Autodesk Inventor part; units mm, degrees
ref_plane "YZ Plane" through (0, 0, 0) normal (1, 0, 0) x (0, 1, 0)
ref_plane "XZ Plane" through (0, 0, 0) normal (0, 1, 0) x (-1, 0, 0)
ref_plane "XY Plane" through (0, 0, 0) normal (0, 0, 1) x (1, 0, 0)
sketch "Sketch9" plane through (0, 0, 0) normal (0, 1, 0) x (-1, 0, 0)
  line L0 (25, 25) -> (-25, 25)
  line L1 (-25, 25) -> (-25, -25)
  line L2 (-25, -25) -> (25, -25)
  line L3 (25, -25) -> (25, 25)
  line L4 (25, 25) -> (-25, -25) construction
  line L5 (-25, 25) -> (25, -25) construction
  line L6 (-23, 23) -> (23, 23)
  line L7 (23, 23) -> (23, -23)
  line L8 (23, -23) -> (-23, -23)
  line L9 (-23, -23) -> (-23, 23)
  point P0 (0, 0)
  dimension "d172" = 50
  dimension "d173" = 50
  dimension "d174" = 2
extrude "Extrusion3" add sketch "Sketch9" against normal blind 930
sketch "Sketch10" plane through (0, 0, 0) normal (1, 0, 0) x (0, 1, 0)
  line L0 (0, 25) -> (0, -25) construction
  line L1 (0, 25) -> (-930, 25) construction
  line L2 (-930, -25) -> (-930, 25) construction
  line L3 (0, -25) -> (-930, -25) construction
  line L4 (-925, 8.5) -> (-908, 8.5)
  line L5 (-908, 8.5) -> (-908, -8.5)
  line L6 (-908, -8.5) -> (-925, -8.5)
  line L7 (-925, -8.5) -> (-925, 8.5)
  line L8 (-925, 8.5) -> (-908, -8.5) construction
  line L9 (-908, 8.5) -> (-925, -8.5) construction
  circle A0 centre (-916.5, 0) radius 8.5
  line L10 (0, 25) -> (0, -25)
  point P0 (0, 0)
  point P1 (0, 0)
  point P2 (-930, 0)
  dimension "d177" = 17
  dimension "d178" = 17
  dimension "d191" = 5
extrude "Extrusion4" cut sketch "Sketch10" along normal through all contours A0
pattern_linear "Rectangular Pattern4" count 8 spacing 125 along (0, 1, 0) of "Extrusion4"
properties part number "TKS 3535 FDS WAY tube5" material "Stainless Steel"
Source: CAD feature listing. Evaluate the final solid. Frame: model axes, mm. A direction names the side the tool comes from. Give positions to 0.01 mm unless a question says otherwise; leave off trailing zeros. Loops run counter-clockwise (first coordinate to the right, second up) from the corner with the lowest first, then second, coordinate; pieces in that order, holes last. Notation, with made-up numbers: (68.5, 85.5) -> (122.5, 85.5) arc R8 cw to (122.5, 97.5) -> close; hole circle Ø5 at (14, 37.25). An arc over 180 degrees is marked (long way). Use a Markdown table: item, result. Add a question column.
1) Pull-direction query (Z, two-part tool) for faces 4 (the face through (2, 0, -24)), 5 (the face through (0, -458, 23)), 6 (the face through (0, -458, -25)); classes: +Z half, -Z half, draft (parallel to the pull), parting line (faces both ways), or undercut.
2) Reachability of faces 1 (the face through (24, -550, 0)), 2 (the face through (2, -930, -24)), 3 (the face through (0, -458, -23)) from +Z, -Z, +X, -X, +Y, -Y: full face, straight path, thin tool, end or side. Return the list, or none.
3) Line query: line 1 along Z through (x, y) = (-11, -457); line 2 along Z through (x, y) = (24.25, -416.5). Output: solid intervals per line, ascending. Write a range as [from, to].
4) Section query B-B, the plane y = -273.5. Return the cut outline in (x, z).
5) Section query C-C, the plane y = -666.5. Return the cut outline in (x, z), then the cut area to 3 significant figures.
6) Section query D-D, the plane z = 0. Count the separate pieces of the cut face and the enclosed holes in it, then the cut area to 3 significant figures.
7) Section query A-A, the plane x = -1. Return the cut outline in (y, z), then the cut area to 3 significant figures.
Numbers:
| question | item | result |
|---|---|---|
| 1 | face 4 | draft |
| 1 | face 5 | undercut |
| 1 | face 6 | -Z half |
| 2 | face 1 | +X |
| 2 | face 2 | +Z, -Z, +X, -X, -Y |
| 2 | face 3 | +Y, -Y |
| 3 | line 1 | z = [-25, -23], [23, 25] |
| 3 | line 2 | z = [-25, -8.5], [8.5, 25] |
| 4 | outline | (-25, -25) -> (25, -25) -> (25, 25) -> (-25, 25) -> close; hole (-23, -23) -> (23, -23) -> (23, 23) -> (-23, 23) -> close |
| 5 | outline | (-25, -25) -> (25, -25) -> (25, -8.5) -> (23, -8.5) -> (23, -23) -> (-23, -23) -> (-23, 23) -> (23, 23) -> (23, 8.5) -> (25, 8.5) -> (25, 25) -> (-25, 25) -> close |
| 5 | area | 350 mm2 |
| 6 | separate pieces | 10 |
| 6 | enclosed holes | 0 |
| 6 | area | 3,450 mm2 |
| 7 | outline | (-930, -25) -> (0, -25) -> (0, -23) -> (-930, -23) -> close; (-930, 23) -> (0, 23) -> (0, 25) -> (-930, 25) -> close |
| 7 | area | 3,720 mm2 |
